from build123d import *

# Parameters (mm, degrees)
SKETCH1_W                   = 2.54
SKETCH1_H                   = 2.54
BOSS_EXTRUDE1_DEPTH         = 5
SKETCH2_W                   = 0.65
SKETCH2_H                   = 0.65
BOSS_EXTRUDE2_DEPTH         = 3
CHAMFER1_SIZE               = 0.15
CHAMFER1_SIZE2              = 0.259807621
SKETCH3_W                   = 0.8
SKETCH3_H                   = 0.8
CUT_EXTRUDE1_DEPTH          = 3
CHAMFER2_SIZE               = 0.6
LPATTERN1_COUNT             = 6
LPATTERN1_PITCH             = 2.54
CHAMFER1_OF_LPATTERN1_SIZE2 = 0.15
CHAMFER1_OF_LPATTERN1_SIZE  = 0.259807621
CHAMFER2_OF_LPATTERN1_SIZE  = 0.6


with BuildPart() as part:
    # Sketch1 → Boss-Extrude1 (new body)
    with BuildSketch(Plane(origin=(0, 0, 0), x_dir=(1, 0, 0), z_dir=(0, 1, 0))):
        Rectangle(SKETCH1_W, SKETCH1_H)
    boss_extrude1 = extrude(amount=BOSS_EXTRUDE1_DEPTH)

    # Sketch2 → Boss-Extrude2 (add)
    with BuildSketch(Plane.XZ):
        Rectangle(SKETCH2_W, SKETCH2_H)
    boss_extrude2 = extrude(amount=BOSS_EXTRUDE2_DEPTH)

    # Chamfer1
    chamfer1_edges = [part.edges().sort_by_distance(p)[0] for p in [
        (0.325, -3, 0),
        (0, -3, 0.325),
        (-0.325, -3, 0),
        (0, -3, -0.325),
    ]]
    chamfer1_side = [part.faces().sort_by_distance(p)[0] for p in [
        (0, -3, 0),
    ]]
    chamfer(chamfer1_edges, length=CHAMFER1_SIZE, length2=CHAMFER1_SIZE2, reference=chamfer1_side[0])

    # Sketch3 → Cut-Extrude1 (cut)
    with BuildSketch(Plane(origin=(0, 5, 0), x_dir=(1, 0, 0), z_dir=(0, 1, 0))):
        Rectangle(SKETCH3_W, SKETCH3_H)
    cut_extrude1 = extrude(amount=-CUT_EXTRUDE1_DEPTH, mode=Mode.SUBTRACT)

    # Chamfer2
    chamfer2_edges = [part.edges().sort_by_distance(p)[0] for p in [
        (0.4, 5, 0),
        (0, 5, -0.4),
        (-0.4, 5, 0),
        (0, 5, 0.4),
    ]]
    chamfer(chamfer2_edges, length=CHAMFER2_SIZE)

    # LPattern1: Boss-Extrude1, Boss-Extrude2, Cut-Extrude1 ×6
    with Locations(*[(i * LPATTERN1_PITCH, 0, 0) for i in range(1, LPATTERN1_COUNT)]):
        add(boss_extrude1)
        add(boss_extrude2)
        add(cut_extrude1, mode=Mode.SUBTRACT)

    # Chamfer1 of LPattern1
    chamfer1_of_lpattern1_edges = [part.edges().sort_by_distance(p)[0] for p in [
        (2.865, -3, 0),
        (2.54, -3, 0.325),
        (2.215, -3, 0),
        (2.54, -3, -0.325),
        (5.405, -3, 0),
        (5.08, -3, 0.325),
        (4.755, -3, 0),
        (5.08, -3, -0.325),
        (7.945, -3, 0),
        (7.62, -3, 0.325),
        (7.295, -3, 0),
        (7.62, -3, -0.325),
        (10.485, -3, 0),
        (10.16, -3, 0.325),
        (9.835, -3, 0),
        (10.16, -3, -0.325),
        (13.025, -3, 0),
        (12.7, -3, 0.325),
        (12.375, -3, 0),
        (12.7, -3, -0.325),
    ]]
    chamfer(chamfer1_of_lpattern1_edges, length=CHAMFER1_OF_LPATTERN1_SIZE, length2=CHAMFER1_OF_LPATTERN1_SIZE2)

    # Chamfer2 of LPattern1
    chamfer2_of_lpattern1_edges = [part.edges().sort_by_distance(p)[0] for p in [
        (2.94, 5, 0),
        (2.54, 5, -0.4),
        (2.14, 5, 0),
        (2.54, 5, 0.4),
        (5.48, 5, 0),
        (5.08, 5, -0.4),
        (4.68, 5, 0),
        (5.08, 5, 0.4),
        (8.02, 5, 0),
        (7.62, 5, -0.4),
        (7.22, 5, 0),
        (7.62, 5, 0.4),
        (10.56, 5, 0),
        (10.16, 5, -0.4),
        (9.76, 5, 0),
        (10.16, 5, 0.4),
        (13.1, 5, 0),
        (12.7, 5, -0.4),
        (12.3, 5, 0),
        (12.7, 5, 0.4),
    ]]
    chamfer(chamfer2_of_lpattern1_edges, length=CHAMFER2_OF_LPATTERN1_SIZE)


solid = part.part
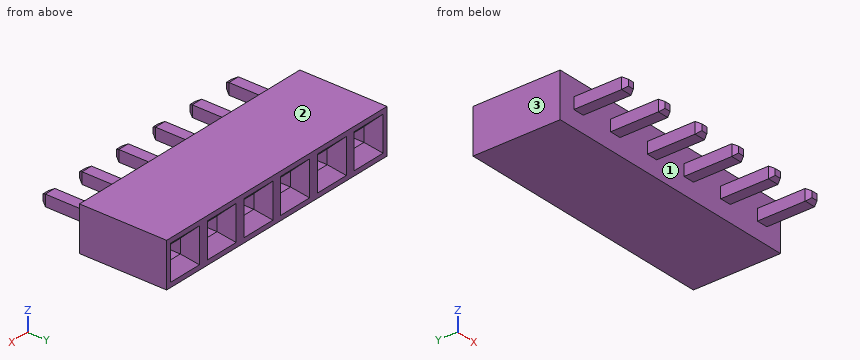
Work out the finished part from the listing and answer in its coordinate system (mm). Face numbers are marked on the shaded views. Give positions to 0.01 mm unless a question says otherwise; leave off trailing zeros. Loops run counter-clockwise (first coordinate to the right, second up) from the corner with the lowest first, then second, coordinate; pieces in that order, holes last. Notation, with made-up numbers: (80, 26) -> (106, 26) arc R23 ccw to (106, 61) -> close; hole circle Ø2 at (65.5, -13.75). An arc over 180 degrees is marked (long way). Use a Markdown table: item, result. Add a question column.
1) Consider line 1 along Y through (x, z) = (5, 1.1); line 2 along Z through (x, y) = (10, 3); line 3 along Z through (x, y) = (10.25, -1) (3 decimals). Determine where each line is inside the solid, lowest interval first.
2) The part is cut by section D-D, the plane z = -0.75. Determine the outline of the cut face in (x, y).
3) The part is cut by section A-A, the plane y = -0.75. Determine the outline of the cut face in (x, z) (3 decimals).
4) The part is cut by section C-C, the plane y = 2.75. Determine the outline of the cut face in (x, z).
5) For a pull along X with two mould halves and no side action, classify the marked faces 1, 2 and 3 as +X half, -X half, draft (parallel to the pull), parting line (faces both ways), or undercut.
6) Each of these flat-tipped pins is pushed along its axis until it touches: P1, Ø0.5, axis at y = -1, z = 0, coming from the -X side (3 decimals); P2, Ø0.7, axis at x = 12.5, y = -1.5, coming from the -Z side (3 decimals). Where does it stop, or does it pass through?
7) The part is cut by section B-B, the plane x = 0. Determine the outline of the cut face in (y, z) (3 decimals), plus the area to 3 significant figures.
Reported:
| question | item | result |
|---|---|---|
| 1 | line 1 | y = 0 to 5 |
| 1 | line 2 | z = -1.27 to -0.4, 0.4 to 1.27 |
| 1 | line 3 | z = -0.325 to 0.325 |
| 2 | outline | (-1.27, 0) -> (13.97, 0) -> (13.97, 5) -> (13.7, 5) -> (13.45, 4.75) -> (11.95, 4.75) -> (11.7, 5) -> (11.16, 5) -> (10.91, 4.75) -> (9.41, 4.75) -> (9.16, 5) -> (8.62, 5) -> (8.37, 4.75) -> (6.87, 4.75) -> (6.62, 5) -> (6.08, 5) -> (5.83, 4.75) -> (4.33, 4.75) -> (4.08, 5) -> (3.54, 5) -> (3.29, 4.75) -> (1.79, 4.75) -> (1.54, 5) -> (1, 5) -> (0.75, 4.75) -> (-0.75, 4.75) -> (-1, 5) -> (-1.27, 5) -> close |
| 3 | outline | (-0.325, -0.325) -> (0.325, -0.325) -> (0.325, 0.325) -> (-0.325, 0.325) -> close; (2.215, -0.325) -> (2.865, -0.325) -> (2.865, 0.325) -> (2.215, 0.325) -> close; (4.755, -0.325) -> (5.405, -0.325) -> (5.405, 0.325) -> (4.755, 0.325) -> close; (7.295, -0.325) -> (7.945, -0.325) -> (7.945, 0.325) -> (7.295, 0.325) -> close; (9.835, -0.325) -> (10.485, -0.325) -> (10.485, 0.325) -> (9.835, 0.325) -> close; (12.375, -0.325) -> (13.025, -0.325) -> (13.025, 0.325) -> (12.375, 0.325) -> close |
| 4 | outline | (-1.27, -1.27) -> (13.97, -1.27) -> (13.97, 1.27) -> (-1.27, 1.27) -> close; hole (-0.4, -0.4) -> (0.4, -0.4) -> (0.4, 0.4) -> (-0.4, 0.4) -> close; hole (2.14, -0.4) -> (2.94, -0.4) -> (2.94, 0.4) -> (2.14, 0.4) -> close; hole (4.68, -0.4) -> (5.48, -0.4) -> (5.48, 0.4) -> (4.68, 0.4) -> close; hole (7.22, -0.4) -> (8.02, -0.4) -> (8.02, 0.4) -> (7.22, 0.4) -> close; hole (9.76, -0.4) -> (10.56, -0.4) -> (10.56, 0.4) -> (9.76, 0.4) -> close; hole (12.3, -0.4) -> (13.1, -0.4) -> (13.1, 0.4) -> (12.3, 0.4) -> close |
| 5 | face 1 | undercut |
| 5 | face 2 | draft |
| 5 | face 3 | -X half |
| 6 | P1 | stops at x = -0.325 |
| 6 | P2 | stops at z = -0.325 |
| 7 | outline | (-3, -0.175) -> (-2.74, -0.325) -> (0, -0.325) -> (0, -1.27) -> (5, -1.27) -> (5, -1) -> (4.4, -0.4) -> (2, -0.4) -> (2, 0.4) -> (4.4, 0.4) -> (5, 1) -> (5, 1.27) -> (0, 1.27) -> (0, 0.325) -> (-2.74, 0.325) -> (-3, 0.175) -> close |
| 7 | area | 11.9 mm^2 |
